Part model, mm, in its own coordinate system. Give positions to 0.01 mm unless a question says otherwise; leave off trailing zeros. Order: outer loops, then holes, each group sorted by start corner. A loop starts at its lowest first (then second) coordinate and runs counter-clockwise, first axis right, second up. Notation, with made-up numbers: (33.5, -24) -> (44.5, -24) arc R11 ccw to (44.5, -12) -> close; hole circle Ø5 at (40, 44). An arc over 180 degrees is marked (long way). Write item = value, one per line. Start each with the question number.
(1) Saw through at A-A, the plane z = -0.1. List the corners of the cut face in (x, y) (3 decimals), then the cut area to 3 significant figures.
(2) Saw through at B-B, the plane x = 6.5. List the corners of the cut face in (y, z).
(3) Saw through at C-C, the plane y = 1.85. List the corners of the cut face in (x, z).
(4) Probe line 1 along Y through (x, z) = (6.75, 0.1); line 2 along X through (y, z) = (4, -0.1) (3 decimals); line 3 along X through (y, z) = (2.7, 0.1). List the from-to ranges inside material, lowest first. Write a range as from..to.
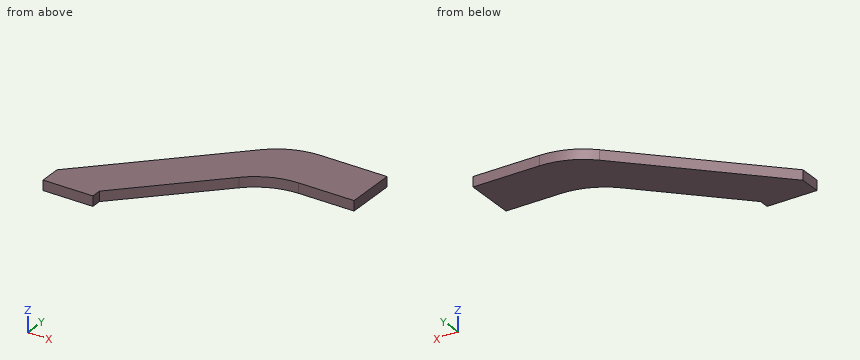
from build123d import *

# Parameters (mm, degrees)
BOSS_EXTRUDE1_DEPTH = 0.15
FILLET1_R           = 2


with BuildPart() as part:
    # Sketch1 → Boss-Extrude1 (new, symmetric)
    with BuildSketch(Plane.XY):
        Polygon((0, 0), (1.5, 0), (1.5, 0.3), (4.611269837, 3.411269837), (7.105, 3.411269837), (7.105, 4.911269837), (4.272792206, 4.911269837), (0, 0.638477631), align=None)
    extrude(amount=BOSS_EXTRUDE1_DEPTH, both=True)

    # Fillet1
    fillet1_edges = [part.edges().sort_by_distance(p)[0] for p in [
        (4.272792206, 4.911269837, 0),
        (4.611269837, 3.411269837, 0),
    ]]
    fillet(fillet1_edges, radius=FILLET1_R)


solid = part.part
Results list:
q1.outline = (0, 0) -> (1.5, 0) -> (1.5, 0.3) -> (4.025, 2.825) arc R2 cw to (5.44, 3.411) -> (7.105, 3.411) -> (7.105, 4.911) -> (5.101, 4.911) arc R2 ccw to (3.687, 4.325) -> (0, 0.638) -> close
q1.area = 11.5 mm^2
q2.outline = (3.41, -0.15) -> (4.91, -0.15) -> (4.91, 0.15) -> (3.41, 0.15) -> close
q3.outline = (1.21, -0.15) -> (3.05, -0.15) -> (3.05, 0.15) -> (1.21, 0.15) -> close
q4.line_1 = 3.41..4.91
q4.line_2 = 3.362..7.105
q4.line_3 = 2.06..3.9
